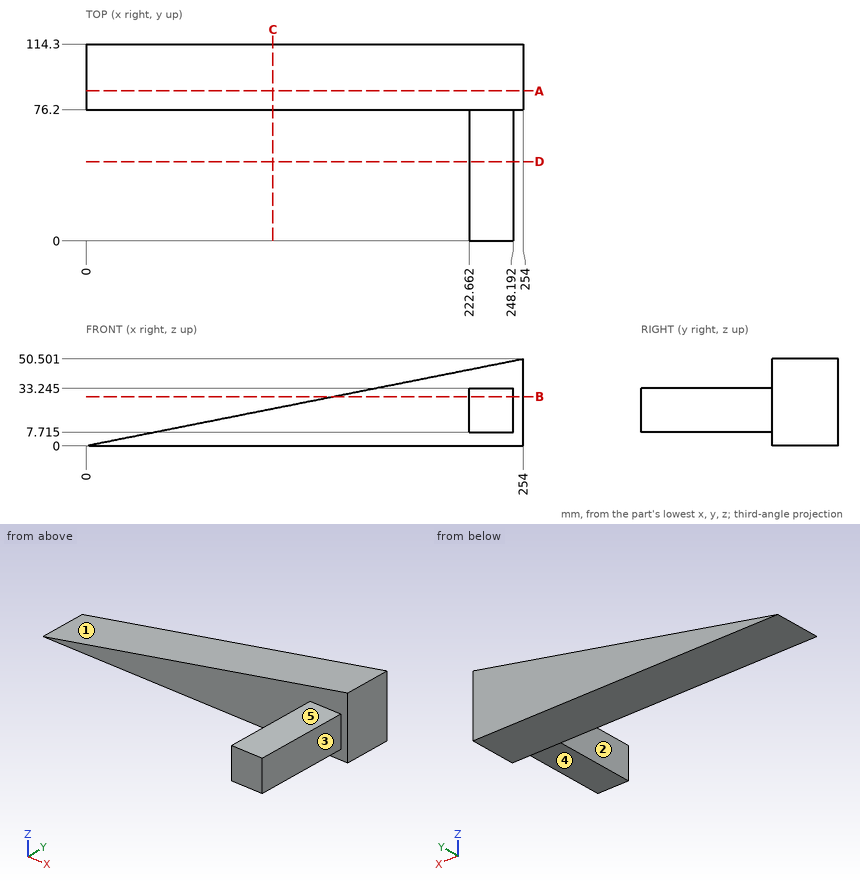
The figure shows three views and two pictorial views of one solid part (mm, origin at its lowest corner). Answer the questions. A direction names the side the tool comes from. Round coordinates to 2 decimals unless told otherwise and drop trailing zeros. Write each loop counter-clockwise with the first axis right and the second up, starting at its lowest first coordinate (ties: lowest second). Pieces come first, ordered by that corner, then holes. Notation, with made-up numbers: M 40.25,59.5 L 52.25,59.5 A15 cw 52.25,69.5 Z; hole C -26.75,61.25 d5. An arc over 180 degrees is marked long. Write each question's results on one line, items separated by ' | '. Start each with the question number.
(1) Each of these flat-tipped pins is pushed along its axis until it touches: P1, Ø20.5, axis at x = 231.5, y = 32, coming from the +Z side (1 decimal); P2, Ø7.5, axis at x = 236, y = 45, coming from the -Z side (1 decimal); P3, Ø2, axis at x = 136, z = 6, coming from the -Y side. Where does it stop, or does it pass through?
(2) For the marked faces 1, 2, 3, 4 and 5, determine the directions among +Z, -Z, +X, -X, +Y, -Y from which every point of the face is accessible in a straight line to the end or side of a thin tool.
(3) The part is cut by section D-D, the plane y = 46. Write down the section's boundary in (x, z) (1 decimal).
(4) The part is cut by section A-A, the plane y = 87. Write down the section's boundary in (x, z).
(5) The part is cut by section B-B, the plane z = 28.5. Write down the section's boundary in (x, y) (1 decimal), and give its area (3 significant figures).
(6) The part is cut by section C-C, the plane x = 108.5. Write down the section's boundary in (y, z), and give its area (3 significant figures).
(7) Find the intervals of material crossed by line 1 (X direction, y = 56.5, z = 27.5); line 2 (Y direction, x = 57, z = 3.5); line 3 (Z direction, x = 174, y = 94.5) (1 decimal), in increasing order.
Worked answers:
1) P1: stops at z = 33.2 | P2: stops at z = 7.7 | P3: stops at y = 76.2
2) face 1: +Z, -X, +Y, -Y | face 2: +Z, -Z, -X, -Y | face 3: +Z, -Z, +X, -Y | face 4: -Z, +X, -X, -Y | face 5: +Z, +X, -X, -Y
3) outline: M 222.7,7.7 L 248.2,7.7 L 248.2,33.2 L 222.7,33.2 Z
4) outline: M 0,0 L 254,0 L 254,50.5 Z
5) outline: M 143.3,76.2 L 222.7,76.2 L 222.7,0 L 248.2,0 L 248.2,76.2 L 254,76.2 L 254,114.3 L 143.3,114.3 Z | area: 6,160 mm²
6) outline: M 76.2,0 L 114.3,0 L 114.3,21.57 L 76.2,21.57 Z | area: 822 mm²
7) line 1: x = 222.66 to 248.19 | line 2: y = 76.2 to 114.3 | line 3: z = 0 to 34.6
